Verification items for the finished model (mm, model axes). Face numbers are marked on the shaded views. A direction names the side the tool comes from. Round coordinates to 2 decimals unless told otherwise and drop trailing zeros. Write each loop counter-clockwise with the first axis right and the second up, starting at its lowest first coordinate (ties: lowest second). Pieces come first, ordered by that corner, then holes. Notation, with made-up numbers: M 34,4 L 68,4 A21 cw 68,27 Z; hole C 82,38.5 d7. An arc over 180 degrees is marked long. One line per item, written item: value. Start each with the question number.
from build123d import *

# Parameters (mm, degrees)
SKETCH2_W           = 600
SKETCH2_H           = 105
SKETCH2_R           = 50
SKETCH2_R_2         = 37.5
BOSS_EXTRUDE2_DEPTH = 80
SKETCH3_W           = 150
SKETCH3_H           = 105.457586359
BOSS_EXTRUDE3_DEPTH = 80
SKETCH4_R           = 5
BOSS_EXTRUDE4_DEPTH = 120
FILLET1_R           = 10
FILLET3_R           = 50
FILLET4_R           = 50
FILLET5_R           = 50
FILLET6_R           = 50
FILLET7_R           = 50


with BuildPart() as part:
    # Sketch2 → Boss-Extrude2 (new body)
    with BuildSketch(Plane(origin=(0, 0, 0), x_dir=(1, 0, 0), z_dir=(0, 1, 0))):
        Rectangle(SKETCH2_W, SKETCH2_H)
        with Locations((-245, 0)):
            Circle(SKETCH2_R, mode=Mode.SUBTRACT)
        with Locations((245, 0)):
            Circle(SKETCH2_R_2, mode=Mode.SUBTRACT)
    extrude(amount=BOSS_EXTRUDE2_DEPTH)

    # Sketch3 → Boss-Extrude3 (add)
    with BuildSketch(Plane(origin=(0, 80, 0), x_dir=(1, 0, 0), z_dir=(0, 1, 0))):
        with Locations((-225, -0.22879318)):
            Rectangle(SKETCH3_W, SKETCH3_H)
    extrude(amount=BOSS_EXTRUDE3_DEPTH)

    # Sketch4 → Boss-Extrude4 (add)
    with BuildSketch(Plane.XZ.offset(-80)):
        with Locations((-245.135702484, 0)):
            Circle(SKETCH4_R)
    extrude(amount=BOSS_EXTRUDE4_DEPTH)

    # Fillet1
    fillet1_edges = [part.edges().sort_by_distance(p)[0] for p in [
        (-150, 160, 0.22879318),
    ]]
    fillet(fillet1_edges, radius=FILLET1_R)

    # Fillet3
    fillet3_edges = [part.edges().sort_by_distance(p)[0] for p in [
        (300, 40, 52.5),
    ]]
    fillet(fillet3_edges, radius=FILLET3_R)

    # Fillet4
    fillet4_edges = [part.edges().sort_by_distance(p)[0] for p in [
        (300, 40, -52.5),
    ]]
    fillet(fillet4_edges, radius=FILLET4_R)

    # Fillet5
    fillet5_edges = [part.edges().sort_by_distance(p)[0] for p in [
        (-300, 40, 52.5),
    ]]
    fillet(fillet5_edges, radius=FILLET5_R)

    # Fillet6
    fillet6_edges = [part.edges().sort_by_distance(p)[0] for p in [
        (-300, 120, 52.957586359),
    ]]
    fillet(fillet6_edges, radius=FILLET6_R)

    # Fillet7
    fillet7_edges = [part.edges().sort_by_distance(p)[0] for p in [
        (-300, 80, -52.5),
    ]]
    fillet(fillet7_edges, radius=FILLET7_R)


solid = part.part
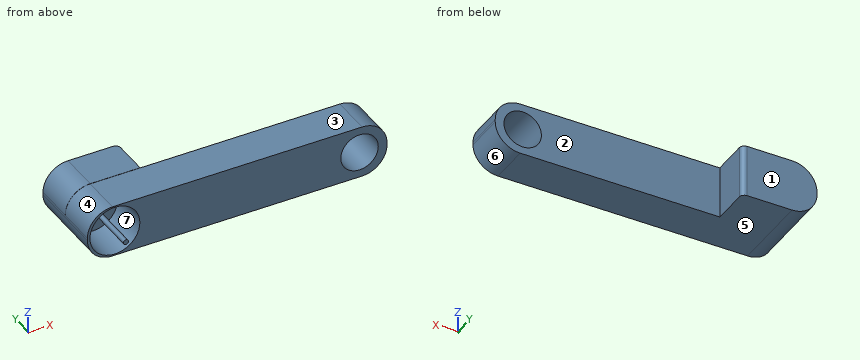
1) Gauge pin test, flat ends, axial feed: pin 1 Ø1.5 at (y, z) = (5.5, -10) entering from -X; pin 2 Ø21 at (y, z) = (107.5, 20) entering from +X; pin 3 Ø25 at (x, z) = (-188.5, 37.5) entering from -Y. Record the tip position at first contact, or that the pin passes through.
2) Mould release check, pull along X, two halves, no side actions. Record for the marked faces 4, 5, 6 and 7: pulls with the +X half, pulls with the -X half, needs draft (parallel to the pull), parting line crosses it, or undercut.
3) Thickness scan on line 1 (Z direction, x = -245, y = 34); line 2 (X direction, y = 41, z = 0.5); line 3 (Z direction, x = 245, y = 50). Record the ranges inside material, lowest first.
4) Cross-section at D-D (x = -63). Record the boundary of the cut face in (y, z), then the cut area to 3 significant figures.
5) Access from +Z, -Z, +X, -X, +Y, -Y to the whole of each face (thin tool, end or side, straight path). Record for the marked faces 1, 2 and 3.
6) Cross-section at C-C (x = 237). Record the boundary of the cut face in (y, z), then the cut area to 3 significant figures.
7) Cross-section at A-A (y = 18). Record the boundary of the cut face in (x, z).
8) Cross-section at B-B (z = 19.5). Record the boundary of the cut face in (x, y).
Results below:
1. pin 1: stops at x = -299.54
1. pin 2: stops at x = -150
1. pin 3: stops at y = 0
2. face 4: pulls with the -X half
2. face 5: needs draft
2. face 6: pulls with the +X half
2. face 7: undercut
3. line 1: z = -52.5 to -50, -5 to 5, 50 to 52.5
3. line 2: x = -300 to -295, -250.11 to -240.16, -195 to 207.5, 282.5 to 300
3. line 3: z = -52.5 to -37.5, 37.5 to 52.5
4. outline: M 0,-52.5 L 80,-52.5 L 80,52.5 L 0,52.5 Z
4. area: 8,400 mm²
5. face 1: +Z, -Z, +X, -X, +Y
5. face 2: +Z, -Z, +X, +Y
5. face 3: +Z, +X, -X, -Y
6. outline: M 0,-52.5 L 80,-52.5 L 80,-36.64 L 0,-36.64 Z; M 0,36.64 L 80,36.64 L 80,52.5 L 0,52.5 Z
6. area: 2,540 mm²
7. outline: M -300,-2.5 A50 ccw -250,-52.5 L 250,-52.5 A50 ccw 300,-2.5 L 300,2.5 A50 ccw 250,52.5 L -250,52.5 A50 ccw -300,2.5 Z; C -245.14,0 d10; hole C -245,0 d100; hole C 245,0 d75
8. outline: M -297.18,80 L -297.02,80 L -297.02,0 L -291.04,0 L -291.04,80 L -198.96,80 L -198.96,0 L 212.97,0 L 212.97,80 L -150,80 L -150,150 A10 ccw -160,160 L -297.18,160 Z; M 277.03,0 L 297.02,0 L 297.02,80 L 277.03,80 Z
